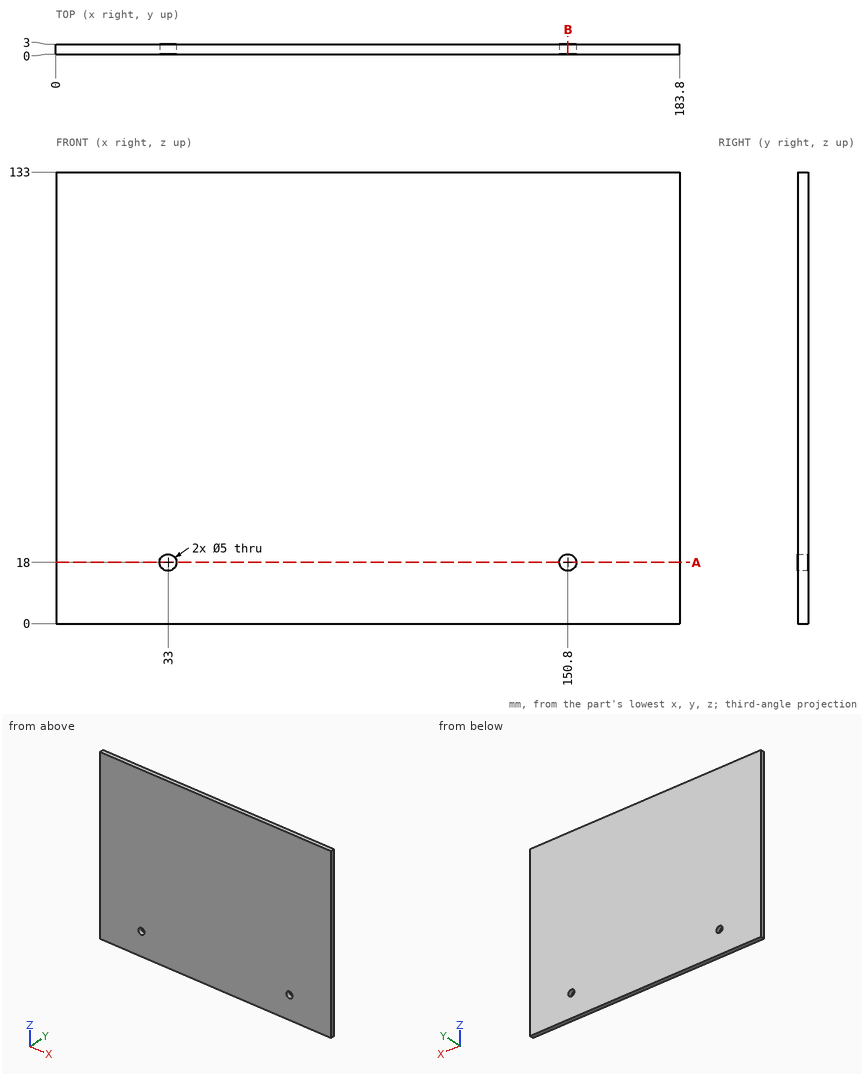
Check sheet for the drawn part. Datum: minimum x, y, z corner. Units: mm. Give positions to 0.01 mm unless a question says otherwise; leave off trailing zeros. Loops run counter-clockwise (first coordinate to the right, second up) from the corner with the lowest first, then second, coordinate; pieces in that order, holes last.
1) Thickness scan on line 1 along X through (y, z) = (0.85, 18); line 2 along Z through (x, y) = (150.8, 1.75). Record the ranges inside material, lowest first.
2) Depth check by flat-ended pin: pin 1 Ø3 at (x, z) = (33, 18) entering from +Y. Enter the tip coordinate at first touch or a pass-through.
3) Sectioned sample at A-A, the plane z = 18. Enter the section's corners in (x, y).
4) Sectioned sample at B-B, the plane x = 150.8. Enter the section's corners in (y, z), then the cut area to 3 significant figures.
Answers:
1. line 1: x = 0 to 30.5, 35.5 to 148.3, 153.3 to 183.8
1. line 2: z = 0 to 15.5, 20.5 to 133
2. pin 1: passes through
3. outline: (0, 0) - (30.5, 0) - (30.5, 3) - (0, 3) - close; (35.5, 0) - (148.3, 0) - (148.3, 3) - (35.5, 3) - close; (153.3, 0) - (183.8, 0) - (183.8, 3) - (153.3, 3) - close
4. outline: (0, 0) - (3, 0) - (3, 15.5) - (0, 15.5) - close; (0, 20.5) - (3, 20.5) - (3, 133) - (0, 133) - close
4. area: 384 mm2
